from build123d import *

# Parameters (mm, degrees)
SKETCH_2_R               = 4
CUT_EXTRUDE_1_DEPTH      = 73.055534139
PATTERN_CIRCULAR_1_COUNT = 6
SKETCH_3_R               = 5
SKETCH_3_R_2             = 25
SKETCH_3_R_3             = 18
EXTRUDE_2_DEPTH          = 12
CHAMFER_1_SIZE           = 3
FILLET_1_R               = 2


with BuildPart() as part:
    # 草圖1 → 旋轉1 (revolve)
    with BuildSketch(Plane(origin=(0, 0, 0), x_dir=(0, 0, -1), z_dir=(1, 0, 0)), mode=Mode.PRIVATE) as revolve_1_sk:
        Polygon((0, 0), (0, 38), (-10, 38), (-10, 18), (-58, 18), (-58, 0), align=None)
    revolve(revolve_1_sk.sketch.rotate(Axis((0, 0, 0), (0, 0, 1)), 90), axis=Axis((0, 0, 0), (0, 0, 1)))

    # 草圖2 → 伸長1 (cut, through all)
    with BuildSketch(Plane.XY.offset(10)):
        with Locations((0, 29)):
            Circle(SKETCH_2_R)
    cut_extrude_1 = extrude(amount=-CUT_EXTRUDE_1_DEPTH, mode=Mode.SUBTRACT)

    # 環狀複製排列1: 伸長1 ×6 about axis
    pattern_circular_1_axis = Axis((0, 0, 0), (0, 0, 1))
    for i in range(1, PATTERN_CIRCULAR_1_COUNT):
        add(cut_extrude_1.rotate(pattern_circular_1_axis, i * 360 / PATTERN_CIRCULAR_1_COUNT), mode=Mode.SUBTRACT)

    # 草圖3 → 伸長2 (add)
    # profile 1 of 3: a face of its own
    with BuildSketch(Plane.XY.offset(58)):
        with BuildLine():
            Line((-11.275939624, 42.105263158), (-23.491540883, 8.552631579))
            ThreePointArc((-23.491540883, 8.552631579), (0, 25), (23.491540883, 8.552631579))
            Line((23.491540883, 8.552631579), (11.275939624, 42.105263158))
            ThreePointArc((11.275939624, 42.105263158), (0, 50), (-11.275939624, 42.105263158))
        make_face()
        with Locations((0, 38)):
            Circle(SKETCH_3_R, mode=Mode.SUBTRACT)
    # profile 2 of 3: a face of its own
    with BuildSketch(Plane.XY.offset(58)):
        Circle(SKETCH_3_R_2)
        with Locations(Location((0, 0, 0), (0, 0, 180))):
            Circle(SKETCH_3_R_3, mode=Mode.SUBTRACT)
    # profile 3 of 3: a face of its own
    with BuildSketch(Plane.XY.offset(58)):
        with BuildLine():
            ThreePointArc((23.491540883, -8.552631579), (0, -25), (-23.491540883, -8.552631579))
            Line((-23.491540883, -8.552631579), (-11.275939624, -42.105263158))
            ThreePointArc((-11.275939624, -42.105263158), (0, -50), (11.275939624, -42.105263158))
            Line((11.275939624, -42.105263158), (23.491540883, -8.552631579))
        make_face()
        with Locations((0, -38)):
            Circle(SKETCH_3_R, mode=Mode.SUBTRACT)
    extrude(amount=-EXTRUDE_2_DEPTH)

    # 草圖4 → 除料-旋轉1 (revolve, cut)
    with BuildSketch(Plane(origin=(0, 0, 0), x_dir=(0, 0, -1), z_dir=(1, 0, 0)), mode=Mode.PRIVATE) as cut_revolve_1_sk:
        Polygon((-58, 0), (-58, 13), (-33, 13), (-33, 10), (0, 10), (0, 0), align=None)
    revolve(cut_revolve_1_sk.sketch.rotate(Axis((0, 0, 0), (0, 0, 1)), 90), axis=Axis((0, 0, 0), (0, 0, 1)), mode=Mode.SUBTRACT)

    # 導角1
    chamfer_1_edges = [part.edges().sort_by_distance(p)[0] for p in [
        (13, 0, 58),
    ]]
    chamfer(chamfer_1_edges, length=CHAMFER_1_SIZE)

    # 圓角1
    fillet_1_edges = [part.edges().sort_by_distance(p)[0] for p in [
        (18, 0, 46),
        (18, 0, 10),
        (38, 0, 10),
    ]]
    fillet(fillet_1_edges, radius=FILLET_1_R)


solid = part.part
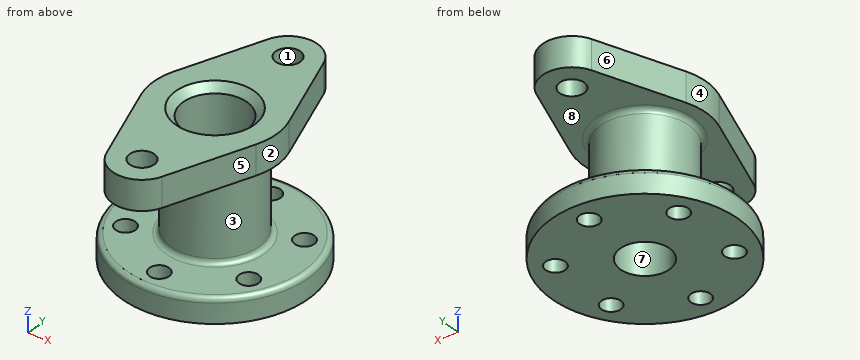
For this review, take the finished solid that the model builds, in its own axes (mm). Face numbers are marked on the shaded views. A direction names the side the tool comes from. Coordinates: 2 decimals unless noted, no trailing zeros. Write each loop counter-clockwise with the first axis right and the second up, starting at its lowest first coordinate (ties: lowest second). Pieces come first, ordered by that corner, then holes. Notation, with made-up numbers: (-11.75, -22) -> (31.25, -22) arc R22 ccw to (31.25, -1) -> close; hole circle Ø4 at (-6, -27). An arc over 180 degrees is marked (long way). Write each question's results on one line, items separated by ' | '. Start each with the question number.
1) Insertion check: pin 1 (4 mm diameter, centred on x = 14.5, z = 33, fed in from -Y); pin 2 (3 mm diameter, centred on x = -9, z = 7, fed in from -Y); pin 3 (6.5 mm diameter, centred on x = 25.11, y = -14.5, fed in from -Z); pin 4 (3 mm diameter, centred on x = -2.5, z = 16, fed in from -Y). Each pin has a flat end and moves straight along its axis. Give the tip position at first contact, or say it passes through.
2) The part is to be moulded in two halves that separate along Y. For the marked faces 6, 7 and 8, say which applies: +Y half, -Y half, draft (parallel to the pull), parting line (faces both ways), or undercut.
3) Wall thickness on L1, parallel to X at y = 14, z = 5; L2, parallel to Y at x = 27.5, z = 9; L3, parallel to X at y = 0.5, z = 5: over which ranges is each line inside the solid? List them lowest first. Write a range as [from, to].
4) Consider section B-B (z = 41). Write out the cut boundary in (x, y).
5) Consider section A-A (y = 0). Write out the cut boundary in (x, z), plus the area to 3 significant figures.
6) For the marked faces 1, 2, 3, 4 and 5, list the 3-axis set-ups (+Z, -Z, +X, -X, +Y, -Y) from which the entire face can be reached by the end or side of a thin tool; tool diameter is ignored.
7) Consider section C-C (x = 0). Give the number of separate pieces and of enclosed holes in the cut face, plus the area to 3 significant figures.
Geometry says:
1) pin 1: y = -12.95 | pin 2: y = -37.25 | pin 3: through | pin 4: y = -17.97
2) face 6: +Y half | face 7: undercut | face 8: draft
3) L1: [-35.33, -29.08], [-21.15, 21.15], [29.08, 35.33] | L2: [-25.84, -17.71], [-11.29, 11.29], [17.71, 25.84] | L3: [-38, -9.99], [9.99, 38]
4) outline: circle Ø36 at (0, 0); hole circle Ø26 at (0, 0)
5) outline: (-38, 0) -> (-10, 0) -> (-10, 33) -> (-13, 33) -> (-13, 55) -> (-16, 58) -> (-25, 58) -> (-25, 46) -> (-20, 46) arc R2 cw to (-18, 44) -> (-18, 12) arc R2 cw to (-20, 10) -> (-36, 10) arc R2 ccw to (-38, 8) -> close; (10, 0) -> (38, 0) -> (38, 8) arc R2 ccw to (36, 10) -> (20, 10) arc R2 cw to (18, 12) -> (18, 44) arc R2 cw to (20, 46) -> (25, 46) -> (25, 58) -> (16, 58) -> (13, 55) -> (13, 33) -> (10, 33) -> close | area: 1,340 mm^2
6) face 1: +Z | face 2: +Z, +X | face 3: none | face 4: +Z, -X | face 5: +Z, +X, -Y
7) separate pieces: 6 | enclosed holes: 0 | area: 1,540 mm^2
